```python
from build123d import *

# Parameters (mm, degrees)
RESSALTO_EXTRUS_O1_DEPTH = 300


with BuildPart() as part:
    # Esboço1 → Ressalto-extrusão1 (new body, symmetric)
    with BuildSketch(Plane.XY):
        with BuildLine():
            Line((-13.1, 8.9), (-14.2, 10))
            Line((-14.2, 10), (-19.6, 10))
            ThreePointArc((-19.6, 10), (-19.882842712, 9.882842712), (-20, 9.6))
            Line((-20, 9.6), (-20, 4.2))
            Line((-20, 4.2), (-18.9, 3.1))
            ThreePointArc((-18.9, 3.1), (-18.617157287, 3.217157287), (-18.5, 3.5))
            Line((-18.5, 3.5), (-18.5, 5.5))
            Line((-18.5, 5.5), (-16.560660172, 5.5))
            Line((-16.560660172, 5.5), (-14.332233047, 3.271572875))
            ThreePointArc((-14.332233047, 3.271572875), (-13.790301169, 2.460514503), (-13.6, 1.503805922))
            Line((-13.6, 1.503805922), (-13.6, 0))
            Line((-13.6, 0), (-13.6, -1.503805922))
            ThreePointArc((-13.6, -1.503805922), (-13.790301169, -2.460514503), (-14.332233047, -3.271572875))
            Line((-14.332233047, -3.271572875), (-16.560660172, -5.5))
            Line((-16.560660172, -5.5), (-18.5, -5.5))
            Line((-18.5, -5.5), (-18.5, -3.5))
            ThreePointArc((-18.5, -3.5), (-18.617157287, -3.217157288), (-18.9, -3.1))
            Line((-18.9, -3.1), (-20, -4.2))
            Line((-20, -4.2), (-20, -9.6))
            ThreePointArc((-20, -9.6), (-19.882842712, -9.882842712), (-19.6, -10))
            Line((-19.6, -10), (-14.2, -10))
            Line((-14.2, -10), (-13.1, -8.9))
            ThreePointArc((-13.1, -8.9), (-13.217157287, -8.617157288), (-13.5, -8.5))
            Line((-13.5, -8.5), (-15.5, -8.5))
            Line((-15.5, -8.5), (-15.5, -6.560660172))
            Line((-15.5, -6.560660172), (-13.271572875, -4.332233047))
            ThreePointArc((-13.271572875, -4.332233047), (-12.460514503, -3.790301169), (-11.503805922, -3.6))
            Line((-11.503805922, -3.6), (-10, -3.6))
            Line((-10, -3.6), (-8.496194078, -3.6))
            ThreePointArc((-8.496194078, -3.6), (-7.539485497, -3.790301169), (-6.728427125, -4.332233047))
            Line((-6.728427125, -4.332233047), (-4.5, -6.560660172))
            Line((-4.5, -6.560660172), (-4.5, -8.5))
            Line((-4.5, -8.5), (-6.5, -8.5))
            ThreePointArc((-6.5, -8.5), (-6.782842712, -8.617157288), (-6.9, -8.9))
            Line((-6.9, -8.9), (-5.8, -10))
            Line((-5.8, -10), (5.8, -10))
            Line((5.8, -10), (6.9, -8.9))
            ThreePointArc((6.9, -8.9), (6.782842712, -8.617157288), (6.5, -8.5))
            Line((6.5, -8.5), (4.5, -8.5))
            Line((4.5, -8.5), (4.5, -6.560660172))
            Line((4.5, -6.560660172), (6.728427125, -4.332233047))
            ThreePointArc((6.728427125, -4.332233047), (7.539485497, -3.790301169), (8.496194078, -3.6))
            Line((8.496194078, -3.6), (10, -3.6))
            Line((10, -3.6), (11.503805922, -3.6))
            ThreePointArc((11.503805922, -3.6), (12.460514503, -3.790301169), (13.271572875, -4.332233047))
            Line((13.271572875, -4.332233047), (15.5, -6.560660172))
            Line((15.5, -6.560660172), (15.5, -8.5))
            Line((15.5, -8.5), (13.5, -8.5))
            ThreePointArc((13.5, -8.5), (13.217157287, -8.617157288), (13.1, -8.9))
            Line((13.1, -8.9), (14.2, -10))
            Line((14.2, -10), (19.6, -10))
            ThreePointArc((19.6, -10), (19.882842712, -9.882842712), (20, -9.6))
            Line((20, -9.6), (20, -4.2))
            Line((20, -4.2), (18.9, -3.1))
            ThreePointArc((18.9, -3.1), (18.617157287, -3.217157288), (18.5, -3.5))
            Line((18.5, -3.5), (18.5, -5.5))
            Line((18.5, -5.5), (16.560660172, -5.5))
            Line((16.560660172, -5.5), (14.332233047, -3.271572875))
            ThreePointArc((14.332233047, -3.271572875), (13.790301169, -2.460514503), (13.6, -1.503805922))
            Line((13.6, -1.503805922), (13.6, 0))
            Line((13.6, 0), (13.6, 1.503805922))
            ThreePointArc((13.6, 1.503805922), (13.790301169, 2.460514503), (14.332233047, 3.271572875))
            Line((14.332233047, 3.271572875), (16.560660172, 5.5))
            Line((16.560660172, 5.5), (18.5, 5.5))
            Line((18.5, 5.5), (18.5, 3.5))
            ThreePointArc((18.5, 3.5), (18.617157287, 3.217157287), (18.9, 3.1))
            Line((18.9, 3.1), (20, 4.2))
            Line((20, 4.2), (20, 9.6))
            ThreePointArc((20, 9.6), (19.882842712, 9.882842712), (19.6, 10))
            Line((19.6, 10), (14.2, 10))
            Line((14.2, 10), (13.1, 8.9))
            ThreePointArc((13.1, 8.9), (13.217157287, 8.617157287), (13.5, 8.5))
            Line((13.5, 8.5), (15.5, 8.5))
            Line((15.5, 8.5), (15.5, 6.560660172))
            Line((15.5, 6.560660172), (13.271572875, 4.332233047))
            ThreePointArc((13.271572875, 4.332233047), (12.460514503, 3.790301169), (11.503805922, 3.6))
            Line((11.503805922, 3.6), (10, 3.6))
            Line((10, 3.6), (8.496194078, 3.6))
            ThreePointArc((8.496194078, 3.6), (7.539485497, 3.790301169), (6.728427125, 4.332233047))
            Line((6.728427125, 4.332233047), (4.5, 6.560660172))
            Line((4.5, 6.560660172), (4.5, 8.5))
            Line((4.5, 8.5), (6.5, 8.5))
            ThreePointArc((6.5, 8.5), (6.782842712, 8.617157288), (6.9, 8.9))
            Line((6.9, 8.9), (5.8, 10))
            Line((5.8, 10), (-5.8, 10))
            Line((-5.8, 10), (-6.9, 8.9))
            ThreePointArc((-6.9, 8.9), (-6.782842712, 8.617157288), (-6.5, 8.5))
            Line((-6.5, 8.5), (-4.5, 8.5))
            Line((-4.5, 8.5), (-4.5, 6.560660172))
            Line((-4.5, 6.560660172), (-6.728427125, 4.332233047))
            ThreePointArc((-6.728427125, 4.332233047), (-7.539485497, 3.790301169), (-8.496194078, 3.6))
            Line((-8.496194078, 3.6), (-10, 3.6))
            Line((-10, 3.6), (-11.503805922, 3.6))
            ThreePointArc((-11.503805922, 3.6), (-12.460514503, 3.790301169), (-13.271572875, 4.332233047))
            Line((-13.271572875, 4.332233047), (-15.5, 6.560660172))
            Line((-15.5, 6.560660172), (-15.5, 8.5))
            Line((-15.5, 8.5), (-13.5, 8.5))
            ThreePointArc((-13.5, 8.5), (-13.217157287, 8.617157287), (-13.1, 8.9))
        make_face()
        with BuildLine():
            Line((-3, 8.5), (3, 8.5))
            Line((3, 8.5), (3, 6.105025253))
            ThreePointArc((3, 6.105025253), (3.030448187, 5.95195188), (3.117157288, 5.822182541))
            Line((3.117157288, 5.822182541), (5.667766953, 3.271572875))
            ThreePointArc((5.667766953, 3.271572875), (6.209698831, 2.460514503), (6.4, 1.503805922))
            Line((6.4, 1.503805922), (6.4, 0))
            Line((6.4, 0), (6.4, -1.503805922))
            ThreePointArc((6.4, -1.503805922), (6.209698831, -2.460514503), (5.667766953, -3.271572875))
            Line((5.667766953, -3.271572875), (3.117157288, -5.822182541))
            ThreePointArc((3.117157288, -5.822182541), (3.030448187, -5.95195188), (3, -6.105025253))
            Line((3, -6.105025253), (3, -8.5))
            Line((3, -8.5), (-3, -8.5))
            Line((-3, -8.5), (-3, -6.105025253))
            ThreePointArc((-3, -6.105025253), (-3.030448187, -5.95195188), (-3.117157288, -5.822182541))
            Line((-3.117157288, -5.822182541), (-5.667766953, -3.271572875))
            ThreePointArc((-5.667766953, -3.271572875), (-6.209698831, -2.460514503), (-6.4, -1.503805922))
            Line((-6.4, -1.503805922), (-6.4, 0))
            Line((-6.4, 0), (-6.4, 1.503805922))
            ThreePointArc((-6.4, 1.503805922), (-6.209698831, 2.460514503), (-5.667766953, 3.271572875))
            Line((-5.667766953, 3.271572875), (-3.117157288, 5.822182541))
            ThreePointArc((-3.117157288, 5.822182541), (-3.030448187, 5.95195188), (-3, 6.105025253))
            Line((-3, 6.105025253), (-3, 8.5))
        make_face(mode=Mode.SUBTRACT)
        with BuildLine():
            ThreePointArc((-10, 2.5), (-11.767766953, 1.767766953), (-12.5, 0))
            ThreePointArc((-12.5, 0), (-11.767766953, -1.767766953), (-10, -2.5))
            ThreePointArc((-10, -2.5), (-8.232233047, -1.767766953), (-7.5, 0))
            ThreePointArc((-7.5, 0), (-8.232233047, 1.767766953), (-10, 2.5))
        make_face(mode=Mode.SUBTRACT)
        with BuildLine():
            ThreePointArc((12.5, 0), (11.767766953, -1.767766953), (10, -2.5))
            ThreePointArc((10, -2.5), (8.232233047, -1.767766953), (7.5, 0))
            ThreePointArc((7.5, 0), (8.232233047, 1.767766953), (10, 2.5))
            ThreePointArc((10, 2.5), (11.767766953, 1.767766953), (12.5, 0))
        make_face(mode=Mode.SUBTRACT)
    extrude(amount=RESSALTO_EXTRUS_O1_DEPTH, both=True)


solid = part.part
```
The model under review builds one solid part; all positions refer to its coordinate system, in mm. Round coordinates to 2 decimals unless told otherwise and drop trailing zeros. Use a Markdown table: item, result. Add a question column.
Q1. For probe 1 along Y at (x, z) = (5.5, 138.5); probe 2 along X at (y, z) = (9.25, -268.5); probe 3 along X at (y, z) = (6.5, -48.5), list the stretches that pass through material, from the lowest coordinate up.
Q2. Add section A-A (z = 82). State how many separate pieces and enclosed holes the cut face has, plus the area to 3 significant figures.
Q3. Insertion check: pin 1 Ø0.9 at (y, z) = (0.5, -111) entering from +X; pin 2 Ø3.5 at (y, z) = (-0.5, 145) entering from +X; pin 3 Ø3.5 at (x, z) = (-10.5, -51) entering from -Y; pin 4 Ø12 at (x, y) = (-10.5, 1.5) entering from -Z. Each pin has a flat end and moves straight along its axis. Give the tip position at first contact, or say it passes through.
Worked answers:
| question | item | result |
|---|---|---|
| 1 | probe 1 | -10 to -8.5, -5.56 to -3.44, 3.44 to 5.56, 8.5 to 10 |
| 1 | probe 2 | -20 to -13.45, -6.55 to 6.55, 13.45 to 20 |
| 1 | probe 3 | -20 to -15.44, -4.56 to -3, 3 to 4.56, 15.44 to 20 |
| 2 | separate pieces | 1 |
| 2 | enclosed holes | 3 |
| 2 | area | 269 mm² |
| 3 | pin 1 | x = 13.6 |
| 3 | pin 2 | x = 13.71 |
| 3 | pin 3 | y = -3.71 |
| 3 | pin 4 | z = -300 |
